from build123d import *

# Parameters (mm, degrees)
F1_DEPTH = 5
F2_R     = 25.4
F3_R     = 7.62
F5_D     = 4.4


with BuildPart() as f1:
    # F0 (on Top) → F1 (new body)
    with BuildSketch(Plane.XY):
        Polygon((-40, 80), (-70, 0), (70, 0), (40, 80), align=None)
    extrude(amount=F1_DEPTH)

    # F2
    f2_edges = [f1.edges().sort_by_distance(p)[0] for p in [
        (-40, 80, 2.5),
        (40, 80, 2.5),
    ]]
    fillet(f2_edges, radius=F2_R)

    # F3
    f3_edges = [f1.edges().sort_by_distance(p)[0] for p in [
        (-70, 0, 2.5),
        (70, 0, 2.5),
    ]]
    fillet(f3_edges, radius=F3_R)

    # F5 (through all)
    with Locations(Plane.XY.offset(5)):
        with Locations((-29.5821707696, 70), (29.5821707696, 70), (52.8025653534, 10), (-52.8025653534, 10)):
            Hole(F5_D / 2)


solid = f1.part
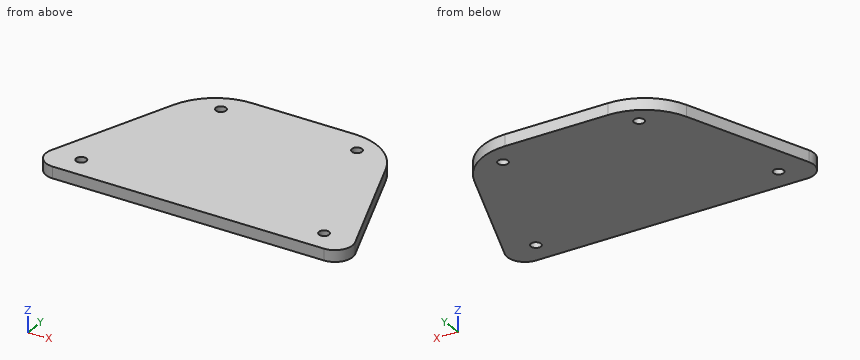
Could you check a few things on this model? Use its own coordinates, in mm. Coordinates: 2 decimals unless noted, no trailing zeros. Order: outer loops, then holes, each group sorted by start corner. A loop starts at its lowest first (then second) coordinate and runs counter-clockwise, first axis right, second up. Notation, with made-up numbers: (45.25, 5) - (100.25, 5) arc R22 cw to (100.25, 26) - close; hole circle Ø6 at (46.25, 35.25). An arc over 180 degrees is marked (long way). Answer in a Markdown table with one row per item. Add a question column.
(1) If we section it at A-A, the plane z = 3.5: Please give me the cut outline in (x, y), then the cut area to 3 significant figures.
(2) I need wall thicknesses on L1, parallel to Y at x = 31, z = 2.3; L2, parallel to Y at x = -30.5, z = 4.25; L3, parallel to Y at x = 22.5, z = 3.7. Which ranges of each line are inside material? Lowest first, please.
(3) If we section it at C-C, the plane x = 56.5: Please give me the cut outline in (y, z).
(4) If we section it at B-B, the plane y = 70: Please give me the cut outline in (x, z).
(5) Will this pin go through, and if not, where does the flat tip stop? pin 1 (1.5 mm diameter, centred on x = -27, z = 4.5, fed in from +Y).
(6) If we section it at D-D, the plane y = 56: Please give me the cut outline in (x, z).
Results are:
| question | item | result |
|---|---|---|
| 1 | outline | (-66.14, 10.3) arc R7.62 ccw to (-59, 0) - (59, 0) arc R7.62 ccw to (66.14, 10.3) - (46.18, 63.52) arc R25.4 ccw to (22.4, 80) - (-22.4, 80) arc R25.4 ccw to (-46.18, 63.52) - close; hole circle Ø4.4 at (-52.8, 10); hole circle Ø4.4 at (-29.58, 70); hole circle Ø4.4 at (29.58, 70); hole circle Ø4.4 at (52.8, 10) |
| 1 | area | 8,570 mm2 |
| 2 | L1 | y = 0 to 68.32, 71.68 to 78.5 |
| 2 | L2 | y = 0 to 68, 72 to 78.67 |
| 2 | L3 | y = 0 to 80 |
| 3 | outline | (0, 0) - (36, 0) - (36, 5) - (0, 5) - close |
| 4 | outline | (-42.6, 0) - (-31.78, 0) - (-31.78, 5) - (-42.6, 5) - close; (-27.38, 0) - (27.38, 0) - (27.38, 5) - (-27.38, 5) - close; (31.78, 0) - (42.6, 0) - (42.6, 5) - (31.78, 5) - close |
| 5 | pin 1 | stops at y = 79.71 |
| 6 | outline | (-49, 0) - (49, 0) - (49, 5) - (-49, 5) - close |
